from build123d import *

# Parameters (mm, degrees)
F0_R     = 15.875
F0_R_2   = 11.25
F1_DEPTH = 38
F2_R     = 4
F4_DEPTH = 15.876


# Not quite as in the source:
# - a fillet or chamfer that OpenCascade refuses, or shapes differently, is made with other operations: its cross-section is extruded or revolved along the edge and cut away or added


with BuildPart() as f1:
    # F0 (on Top) → F1 (new body)
    with BuildSketch(Plane.XY):
        Circle(F0_R)
        Circle(F0_R_2, mode=Mode.SUBTRACT)
    extrude(amount=F1_DEPTH)

    # F3: chamfer of 5 on 2 edges, made by hand

    # F3_s1 → F3_t2 (revolve, cut)
    with BuildSketch(Plane.XZ):
        Polygon((15.875, 33), (10.875, 38), (15.875, 38), align=None)
    revolve(axis=Axis((0, 0, 38), (0, 0, 1)), mode=Mode.SUBTRACT)

    # F3_s3 → F3_t4 (revolve, cut)
    with BuildSketch(Plane.XZ):
        Polygon((15.875, 5), (10.875, 0), (15.875, 0), align=None)
    revolve(axis=Axis((0, 0, 0), (0, 0, 1)), mode=Mode.SUBTRACT)

    # F2 (on Front) → F4 (cut, through all)
    with BuildSketch(Plane.XZ):
        with Locations((7, 19)):
            Circle(F2_R)
        with Locations((-7, 19)):
            Circle(F2_R)
    extrude(amount=-F4_DEPTH, mode=Mode.SUBTRACT)


solid = f1.part
Design review of the part built by this model. Coordinates are the model's own, in mm. Give positions to 0.01 mm unless a question says otherwise; leave off trailing zeros. Loops run counter-clockwise (first coordinate to the right, second up) from the corner with the lowest first, then second, coordinate; pieces in that order, holes last. Notation, with made-up numbers: M -27.75,12.5 L 28.25,12.5 A17 ccw 28.25,43.5 Z; hole C 47,79.25 d5. An arc over 180 degrees is marked long. One line per question, with ' | ' between items. Start each with the question number.
1. To check wall thickness, follow L1, parallel to Y at x = 0, z = 26 (3 decimals); L2, parallel to Z at x = 4, y = 12.5; L3, parallel to Y at x = -10, z = 35. State the ranges of each line that lie inside material, in increasing order.
2. Add section C-C (z = 14). Write out the cut boundary in (x, y) (3 decimals), plus the area to 3 significant figures.
3. Add section A-A (x = 0). Write out the cut boundary in (y, z) (3 decimals), plus the area to 3 significant figures.
4. The part is to be moulded in two halves that separate along Z. For faces 1 (the face through (10.815, 10.357, 20.201)), 2 (the face through (10.945, 3.447, 0.6)), 3 (the face through (-11, 10, 19)), 4 (the face through (10.945, 3.447, 37.4)), say which applies: released by +Z, released by -Z, zero draft, split by the parting line, or undercut.
5. Insertion check: P1, Ø1.5, axis at x = 12.5, z = 8, coming from the -Y side; P2, Ø4, axis at x = 7, z = 32.5, coming from the -Y side; P3, Ø6.5, axis at x = 7, z = 19, coming from the +Y side; P4, Ø13.5, axis at x = 0, y = 0, coming from the +Z side. Each pin has a flat end and moves straight along its axis. Give the tip position at first contact, or say it passes through.
6. Add section D-D (x = 10.5). Give the number of separate pieces and of enclosed holes in the cut face, plus the area to 3 significant figures.
Worked out:
1) L1: y = -15.875 to -11.25, 11.25 to 15.875 | L2: z = 2.25 to 16.35, 21.65 to 35.75 | L3: y = -9.62 to -5.15, 5.15 to 9.62
2) outline: C 0,0 d31.75; hole C 0,0 d22.5 | area: 394 mm²
3) outline: M -15.875,5 L -11.25,0.375 L -11.25,37.625 L -15.875,33 Z; M 11.25,0.375 L 15.875,5 L 15.875,33 L 11.25,37.625 Z | area: 302 mm²
4) face 1: undercut | face 2: released by -Z | face 3: undercut | face 4: released by +Z
5) P1: stops at y = -10.67 | P2: stops at y = -15.07 | P3: stops at y = -4.64 | P4: passes through
6) separate pieces: 3 | enclosed holes: 0 | area: 491 mm²
